```python
from build123d import *

# Parameters (mm, degrees)
SKETCH1_W           = 6
SKETCH1_H           = 6
BOSS_EXTRUDE1_DEPTH = 2.28
SKETCH2_R           = 1.725
CUT_EXTRUDE1_DEPTH  = 1
CUT_EXTRUDE2_DEPTH  = 0.05
CUT_EXTRUDE3_DEPTH  = 1
SKETCH5_R           = 1.625
BOSS_EXTRUDE2_DEPTH = 1.2
CUT_EXTRUDE6_DEPTH  = 1.2
SKETCH7_R           = 0.5
CUT_EXTRUDE7_DEPTH  = 0.5


with BuildPart() as part:
    # Sketch1 → Boss-Extrude1 (new body)
    with BuildSketch(Plane.XY):
        Rectangle(SKETCH1_W, SKETCH1_H)
    extrude(amount=BOSS_EXTRUDE1_DEPTH)

    # Sketch2 → Cut-Extrude1 (cut)
    with BuildSketch(Plane.XY.offset(2.28)):
        with Locations((-0.245, 0.382)):
            Circle(SKETCH2_R)
    extrude(amount=-CUT_EXTRUDE1_DEPTH, mode=Mode.SUBTRACT)

    # Sketch3 → Cut-Extrude2 (cut)
    with BuildSketch(Plane.XY.offset(2.28)):
        with BuildLine():
            Line((0.815660172, -1.385766953), (-2.012766953, 1.442660172))
            ThreePointArc((-2.012766953, 1.442660172), (-2.012766953, 2.149766953), (-1.305660172, 2.149766953))
            Line((-1.305660172, 2.149766953), (1.522766953, -0.678660172))
            ThreePointArc((1.522766953, -0.678660172), (1.522766953, -1.385766953), (0.815660172, -1.385766953))
        make_face()
    extrude(amount=-CUT_EXTRUDE2_DEPTH, mode=Mode.SUBTRACT)

    # Sketch4 → Cut-Extrude3 (cut)
    with BuildSketch(Plane.XY.offset(2.28)):
        with BuildLine():
            Line((-2.45, -2.7), (-2.45, -3))
            Line((-2.45, -3), (-0.95, -3))
            Line((-0.95, -3), (-0.95, -2.7))
            ThreePointArc((-0.95, -2.7), (-1.7, -1.95), (-2.45, -2.7))
        make_face()
    extrude(amount=-CUT_EXTRUDE3_DEPTH, mode=Mode.SUBTRACT)

    # Sketch5 → Boss-Extrude2 (add)
    with BuildSketch(Plane.XY.offset(1.28)):
        with Locations((-0.245, 0.382)):
            Circle(SKETCH5_R)
    extrude(amount=BOSS_EXTRUDE2_DEPTH)

    # Sketch6 → Cut-Extrude6 (cut)
    with BuildSketch(Plane.XY.offset(2.48)):
        with BuildLine():
            ThreePointArc((-1.897587238, 0.051650147), (-1.801997597, -0.262929521), (-1.647148264, -0.552963022))
            ThreePointArc((-1.647148264, -0.552963022), (-1.498242435, -0.137110013), (-1.897587238, 0.051650147))
        make_face()
        with BuildLine():
            ThreePointArc((0.085349853, 2.034587238), (0.274110013, 1.635242435), (0.689963022, 1.784148264))
            ThreePointArc((0.689963022, 1.784148264), (0.399929521, 1.938997597), (0.085349853, 2.034587238))
        make_face()
        with BuildLine():
            ThreePointArc((1.157148264, 1.316963022), (1.008242435, 0.901110013), (1.407587238, 0.712349853))
            ThreePointArc((1.407587238, 0.712349853), (1.311997597, 1.026929521), (1.157148264, 1.316963022))
        make_face()
        with BuildLine():
            ThreePointArc((1.407587238, 0.051650147), (1.008242435, -0.137110013), (1.157148264, -0.552963022))
            ThreePointArc((1.157148264, -0.552963022), (1.311997597, -0.262929521), (1.407587238, 0.051650147))
        make_face()
        with BuildLine():
            ThreePointArc((0.689963022, -1.020148264), (0.274110013, -0.871242435), (0.085349853, -1.270587238))
            ThreePointArc((0.085349853, -1.270587238), (0.399929521, -1.174997597), (0.689963022, -1.020148264))
        make_face()
        with BuildLine():
            ThreePointArc((-0.575349853, -1.270587238), (-0.764110013, -0.871242435), (-1.179963022, -1.020148264))
            ThreePointArc((-1.179963022, -1.020148264), (-0.889929521, -1.174997597), (-0.575349853, -1.270587238))
        make_face()
        with BuildLine():
            ThreePointArc((-1.897587238, 0.712349853), (-1.498242435, 0.901110013), (-1.647148264, 1.316963022))
            ThreePointArc((-1.647148264, 1.316963022), (-1.801997597, 1.026929521), (-1.897587238, 0.712349853))
        make_face()
        with BuildLine():
            ThreePointArc((-1.179963022, 1.784148264), (-0.764110013, 1.635242435), (-0.575349853, 2.034587238))
            ThreePointArc((-0.575349853, 2.034587238), (-0.889929521, 1.938997597), (-1.179963022, 1.784148264))
        make_face()
    extrude(amount=-CUT_EXTRUDE6_DEPTH, mode=Mode.SUBTRACT)

    # Sketch7 → Cut-Extrude7 (cut)
    with BuildSketch(Plane.XY.offset(2.48)):
        with Locations((-0.245, 0.382)):
            Circle(SKETCH7_R)
    extrude(amount=-CUT_EXTRUDE7_DEPTH, mode=Mode.SUBTRACT)


solid = part.part
```
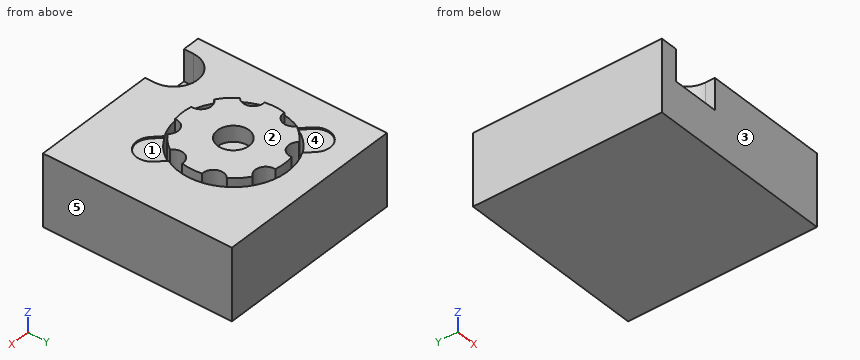
Part model, mm, in its own coordinate system. Face numbers are marked on the shaded views. A direction names the side the tool comes from. Coordinates: 2 decimals unless noted, no trailing zeros. Write each loop counter-clockwise with the first axis right and the second up, starting at its lowest first coordinate (ties: lowest second). Pieces come first, ordered by that corner, then holes.
Item 1: Slice it at A-A (z = 1.8). Write the cut outline in (x, y) (3 decimals), and give its area (3 significant figures).
Item 2: Which spindle directions (+Z, -Z, +X, -X, +Y, -Y) get a long thin tool onto all of the face, cutting with end or side? Do the marked faces 1 and 2. Say none if no direction does.
Item 3: Pin check, flat tip, straight feed: pin 1 (1.2 mm diameter, centred on x = -2, y = -2.5, fed in from +Z). Stop position of the tip, or through.
Item 4: Slice it at B-B (y = 2.6). Write the cut outline in (x, z), and give its area (3 significant figures).
Item 5: Mould opens along Y. For the marked faces 3, 4 and 5 say: released by +Y, released by -Y, zero draft, split by the parting line, or undercut.
Item 6: Probe line 1 (Z direction, x = 0.6, y = 2.1); line 2 (Z direction, x = -1.65, y = -0.55); line 3 (X direction, y = -0.2, z = 1.5). List the from-to ranges inside material, lowest first.
Item 7: Slice it at C-C (x = -0.45). Write the cut outline in (y, z).
Results found:
1. outline: (-3, -3) - (-2.45, -3) - (-2.45, -2.7) arc R0.75 cw to (-0.95, -2.7) - (-0.95, -3) - (3, -3) - (3, 3) - (-3, 3) - close; (-1.839, 0.064) arc R0.329 cw to (-1.597, -0.52) arc R1.625 ccw to (-1.147, -0.97) arc R0.329 cw to (-0.563, -1.212) arc R1.625 ccw to (0.073, -1.212) arc R0.329 cw to (0.657, -0.97) arc R1.625 ccw to (1.107, -0.52) arc R0.329 cw to (1.349, 0.064) arc R1.625 ccw to (1.349, 0.7) arc R0.329 cw to (1.107, 1.284) arc R1.625 ccw to (0.657, 1.734) arc R0.329 cw to (0.073, 1.976) arc R1.625 ccw to (-0.563, 1.976) arc R0.329 cw to (-1.147, 1.734) arc R1.625 ccw to (-1.597, 1.284) arc R0.329 cw to (-1.839, 0.7) arc R1.625 ccw to start; hole circle Ø3.45 at (-0.245, 0.382)
1. area: 32.6 mm2
2. face 1: +Z
2. face 2: +Z, +X, -X, +Y, -Y
3. pin 1: stops at z = 2.28
4. outline: (-3, 0) - (3, 0) - (3, 2.28) - (-3, 2.28) - close
4. area: 13.7 mm2
5. face 3: released by -Y
5. face 4: undercut
5. face 5: zero draft
6. line 1: z = 0 to 2.28
6. line 2: z = 0 to 1.28
6. line 3: x = -3 to -1.87, -1.48 to 0.99, 1.38 to 3
7. outline: (-3, 0) - (3, 0) - (3, 2.28) - (2.09, 2.28) - (2.09, 1.28) - (1.99, 1.28) - (1.99, 2.48) - (0.84, 2.48) - (0.84, 1.98) - (-0.07, 1.98) - (-0.07, 2.48) - (-1.23, 2.48) - (-1.23, 1.28) - (-1.33, 1.28) - (-1.33, 2.28) - (-3, 2.28) - close
